Design review of the part built by this model. Coordinates are the model's own, in mm. A direction names the side the tool comes from. Round coordinates to 2 decimals unless told otherwise and drop trailing zeros. Write each loop counter-clockwise with the first axis right and the second up, starting at its lowest first coordinate (ties: lowest second). Pieces come first, ordered by that corner, then holes. Notation, with made-up numbers: M -21.5,77 L 18.5,77 A22 cw 18.5,83 Z; hole C 73,78.5 d10. An arc over 180 degrees is marked long. Use CSV: the item, a comma, the result in double quotes.
from build123d import *

# Parameters (mm, degrees)
SKETCH_1_W          = 20
SKETCH_1_H          = 10
EXTRUDE_1_DEPTH     = 4
SKETCH_2_W          = 8
SKETCH_2_H          = 10
EXTRUDE_2_DEPTH     = 10
SKETCH_3_R          = 2.499995339
CUT_EXTRUDE_1_DEPTH = 21.420577857
CHAMFER_1_SIZE      = 2


with BuildPart() as part:
    # Эскиз1 → Вытянуть1 (new body)
    with BuildSketch(Plane(origin=(0, 0, 0), x_dir=(1, 0, 0), z_dir=(0, 1, 0))):
        Rectangle(SKETCH_1_W, SKETCH_1_H)
    extrude(amount=EXTRUDE_1_DEPTH)

    # Эскиз2 → Вытянуть2 (add)
    with BuildSketch(Plane(origin=(0, 4, 0), x_dir=(1, 0, 0), z_dir=(0, 1, 0))):
        Rectangle(SKETCH_2_W, SKETCH_2_H)
    extrude(amount=EXTRUDE_2_DEPTH)

    # Эскиз3 → Вырез-Вытянуть1 (cut, through all)
    with BuildSketch(Plane.ZY.offset(4)):
        with Locations((0.128840194, 10)):
            Circle(SKETCH_3_R)
    extrude(amount=-CUT_EXTRUDE_1_DEPTH, mode=Mode.SUBTRACT)

    # Фаска1
    chamfer_1_edges = [part.edges().sort_by_distance(p)[0] for p in [
        (0, 14, -5),
        (0, 14, 5),
    ]]
    chamfer(chamfer_1_edges, length=CHAMFER_1_SIZE)


solid = part.part
1) The part is to be moulded in two halves that separate along Z. For faces 4 (the face through (-0.06, 12.11, 1.47)), 5 (the face through (-10, 2, 0)), 6 (the face through (0, 5, -5)), say which applies: released by +Z, released by -Z, zero draft, split by the parting line, or undercut.
Answers:
face 4,"undercut"
face 5,"zero draft"
face 6,"released by -Z"
2) Machinability: for faces 1 (the face through (0, 13, 4)), 2 (the face through (-4, 7, 0)), 3 (the face through (4, 7, 0)), which of the approach directions +Z, -Z, +X, -X, +Y, -Y give a long, thin tool a straight path to every point of the face, cutting with its end or side? Answer none if there is none.
Answers:
face 1,"+Z, +X, -X, +Y"
face 2,"+Z, -Z, -X, +Y"
face 3,"+Z, -Z, +X, +Y"
3) Add section A-A on x = 1.75. Write out the cut boundary in (y, z), then the cut area to 3 significant figures.
Answers:
outline,"M 0,-5 L 12,-5 L 14,-3 L 14,3 L 12,5 L 0,5 Z; hole C 10,0.13 d5"
area,"116 mm²"
4) Add section C-C on z = -3.5. Write out the cut boundary in (x, y), then the cut area to 3 significant figures.
Answers:
outline,"M -10,0 L 10,0 L 10,4 L 4,4 L 4,13.5 L -4,13.5 L -4,4 L -10,4 Z"
area,"156 mm²"
5) Wall thickness on line 1 along X through (y, z) = (13.25, -1); line 2 along Y through (x, z) = (-5.5, -1.5); line 3 along Y through (x, z) = (-1.5, 0): over which ranges is each line inside the solid? List them lowest first. Write a range as [from, to].
Answers:
line 1,"[-4, 4]"
line 2,"[0, 4]"
line 3,"[0, 7.5], [12.5, 14]"
6) For pin 1 Ø1.5 at (x, z) = (8, 3) entering from -Y; pin 2 Ø4 at (y, z) = (11.5, 1) entering from +X, all flat-tipped, find the tip position at first contact; note any pin that passes through.
Answers:
pin 1,"y = 0"
pin 2,"x = 4"
7) Add section B-B on y = 10. Write out the cut boundary in (x, z).
Answers:
outline,"M -4,-5 L 4,-5 L 4,-2.37 L -4,-2.37 Z; M -4,2.63 L 4,2.63 L 4,5 L -4,5 Z"
8) Add section D-D on z = 1.75. Write out the cut boundary in (x, y), then the cut area to 3 significant figures.
Answers:
outline,"M -10,0 L 10,0 L 10,4 L 4,4 L 4,8.1 L -4,8.1 L -4,4 L -10,4 Z; M -4,11.9 L 4,11.9 L 4,14 L -4,14 Z"
area,"130 mm²"
